```python
from build123d import *

# Parameters (mm, degrees)
SKETCH_1_W             = 140
SKETCH_1_H             = 80
EXTRUDE_1_DEPTH        = 2
SKETCH_2_W             = 5.5
SKETCH_2_H             = 5
SKETCH_2_H_2           = 3
EXTRUDE_2_DEPTH        = 12
SKETCH_3_W             = 30
SKETCH_3_H             = 80
CUT_EXTRUDE_1_DEPTH    = 3
SKETCH_4_W             = 36.4
SKETCH_4_H             = 15.6
SKETCH_4_W_2           = 30.4
SKETCH_4_H_2           = 9.6
EXTRUDE_3_DEPTH        = 18
SKETCH_5_W             = 10
SKETCH_5_H             = 27.4
CUT_EXTRUDE_2_DEPTH    = 20
SKETCH_6_W             = 1.3
SKETCH_6_H             = 9.6
EXTRUDE_4_DEPTH        = 3
SKETCH_8_W             = 10
SKETCH_8_H             = 6.6
CUT_EXTRUDE_3_DEPTH    = 40
PATTERN_LINEAR_1_COUNT = 2
PATTERN_LINEAR_1_PITCH = 40


with BuildPart() as part:
    # 草图1 → 凸台-拉伸1 (new body)
    with BuildSketch(Plane(origin=(0, 0, 0), x_dir=(0, 0, -1), z_dir=(1, 0, 0))):
        Rectangle(SKETCH_1_W, SKETCH_1_H)
    extrude(amount=EXTRUDE_1_DEPTH)

    # 草图2 → 凸台-拉伸2 (add)
    with BuildSketch(Plane(origin=(2, 0, 0), x_dir=(0, 0, -1), z_dir=(1, 0, 0))):
        with Locations((-24.05, -14.7)):
            Rectangle(SKETCH_2_W, SKETCH_2_H)
        with Locations((-52.75, -14.7)):
            Rectangle(SKETCH_2_W, SKETCH_2_H)
        with Locations((-24.05, -21.5)):
            Rectangle(SKETCH_2_W, SKETCH_2_H_2)
        with Locations((-52.75, 18.5)):
            Rectangle(SKETCH_2_W, SKETCH_2_H_2)
        with Locations((-24.05, 25.3)):
            Rectangle(SKETCH_2_W, SKETCH_2_H)
        with Locations((-52.75, -21.5)):
            Rectangle(SKETCH_2_W, SKETCH_2_H_2)
        with Locations((-24.05, 18.5)):
            Rectangle(SKETCH_2_W, SKETCH_2_H_2)
        with Locations((-52.75, 25.3)):
            Rectangle(SKETCH_2_W, SKETCH_2_H)
    extrude(amount=EXTRUDE_2_DEPTH)

    # 草图3 → 切除-拉伸1 (cut)
    with BuildSketch(Plane(origin=(2, 0, 0), x_dir=(0, 0, -1), z_dir=(1, 0, 0))):
        with Locations((55, 0)):
            Rectangle(SKETCH_3_W, SKETCH_3_H)
    extrude(amount=-CUT_EXTRUDE_1_DEPTH, mode=Mode.SUBTRACT)

    # 草图4 → 凸台-拉伸3 (add)
    with BuildSketch(Plane(origin=(2, 0, 0), x_dir=(0, 0, -1), z_dir=(1, 0, 0))):
        with Locations((18.9, -26.7)):
            Rectangle(SKETCH_4_W, SKETCH_4_H)
        with Locations((18.9, -26.7)):
            Rectangle(SKETCH_4_W_2, SKETCH_4_H_2, mode=Mode.SUBTRACT)
    extrude_3 = extrude(amount=EXTRUDE_3_DEPTH)

    # 草图5 → 切除-拉伸2 (cut)
    with BuildSketch(Plane.XZ.offset(34.5)):
        with Locations((7, -18.9)):
            Rectangle(SKETCH_5_W, SKETCH_5_H)
    cut_extrude_2 = extrude(amount=-CUT_EXTRUDE_2_DEPTH, mode=Mode.SUBTRACT)

    # 草图6 → 凸台-拉伸4 (add)
    with BuildSketch(Plane(origin=(2, 0, 0), x_dir=(0, 0, -1), z_dir=(1, 0, 0))):
        with Locations((4.35, -26.7)):
            Rectangle(SKETCH_6_W, SKETCH_6_H)
        with Locations((33.45, -26.7)):
            Rectangle(SKETCH_6_W, SKETCH_6_H)
    extrude_4 = extrude(amount=EXTRUDE_4_DEPTH)

    # 草图8 → 切除-拉伸3 (cut)
    with BuildSketch(Plane(origin=(0, 0, -37.1), x_dir=(-1, 0, 0), z_dir=(0, 0, -1))):
        with Locations((-7, -26.7)):
            Rectangle(SKETCH_8_W, SKETCH_8_H)
    cut_extrude_3 = extrude(amount=-CUT_EXTRUDE_3_DEPTH, mode=Mode.SUBTRACT)

    # 阵列(线性)1: 凸台-拉伸3, 切除-拉伸2, 凸台-拉伸4, 切除-拉伸3 ×2
    with Locations(*[(0, i * PATTERN_LINEAR_1_PITCH, 0) for i in range(1, PATTERN_LINEAR_1_COUNT)]):
        add(extrude_3)
        add(cut_extrude_2, mode=Mode.SUBTRACT)
        add(extrude_4)
        add(cut_extrude_3, mode=Mode.SUBTRACT)


solid = part.part
```
The listing builds one solid part. Answer for the finished solid, in the listing's coordinates (mm). A direction names the side the tool comes from. Round coordinates to 2 decimals unless told otherwise and drop trailing zeros. Order: outer loops, then holes, each group sorted by start corner. A loop starts at its lowest first (then second) coordinate and runs counter-clockwise, first axis right, second up. Notation, with made-up numbers: (16.5, 47) -> (32.5, 47) arc R10 ccw to (32.5, 64) -> close; hole circle Ø9 at (68, 27). An arc over 180 degrees is marked (long way). Answer as CSV lines item,"result".
Q1. Given pin 1 (8 mm diameter, centred on x = 10.5, y = -23, fed in from -Z); pin 2 (5 mm diameter, centred on x = 6.5, y = 2, fed in from +Z); pin 3 (6 mm diameter, centred on x = 5.5, z = 53.5, fed in from +Y); pin 4 (6 mm diameter, centred on x = 7.5, y = -20.5, fed in from +Z), each flat-ended and moving along its own axis, determine where each tip first touches the part or whether it passes through.
Computed values:
pin 1,"stops at z = -37.1"
pin 2,"passes through"
pin 3,"stops at y = 27.8"
pin 4,"stops at z = 55.5"
Q2. Which of the six approach directions +Z, -Z, +X, -X, +Y, -Y give full straight-line access (tool end or side, diameter ignored) to faces 4 (the flat face through (8, 22.8, 53)), 5 (the flat face through (14, 19, 53)), 6 (the flat face through (7, 16.6, -2))?
Computed values:
face 4,"+Z, -Z, +X"
face 5,"+Z, +X, +Y, -Y"
face 6,"+Z, -Z"
Q3. For a pull along Y with two mould halves and no side action, classify faces 1 (the flat face through (8, -15, 26.8)), 2 (the flat face through (7, -23.4, -35)), 3 (the flat face through (15, -34.5, -19)) as +Y half, -Y half, draft (parallel to the pull), parting line (faces both ways), or undercut.
Computed values:
face 1,"draft"
face 2,"undercut"
face 3,"-Y half"
Q4. A cutting plane is placed at B-B on z = -24. Determine the outline of the cut face in (x, y).
Computed values:
outline,"(0, -40) -> (2, -40) -> (2, 40) -> (0, 40) -> close; (12, -34.5) -> (20, -34.5) -> (20, -31.5) -> (12, -31.5) -> close; (12, -21.9) -> (20, -21.9) -> (20, -18.9) -> (12, -18.9) -> close; (12, 5.5) -> (20, 5.5) -> (20, 8.5) -> (12, 8.5) -> close; (12, 18.1) -> (20, 18.1) -> (20, 21.1) -> (12, 21.1) -> close"
Q5. A cutting plane is placed at A-A on x = 17.25. Determine the outline of the cut face in (y, z).
Computed values:
outline,"(-34.5, -37.1) -> (-18.9, -37.1) -> (-18.9, -0.7) -> (-34.5, -0.7) -> close; (5.5, -37.1) -> (21.1, -37.1) -> (21.1, -0.7) -> (5.5, -0.7) -> close; hole (-31.5, -34.1) -> (-21.9, -34.1) -> (-21.9, -3.7) -> (-31.5, -3.7) -> close; hole (8.5, -34.1) -> (18.1, -34.1) -> (18.1, -3.7) -> (8.5, -3.7) -> close"
Q6. A cutting plane is placed at C-C on y = 1.5. Determine the outline of the cut face in (x, z), plus the area to 3 significant figures.
Computed values:
outline,"(0, -40) -> (2, -40) -> (2, 70) -> (0, 70) -> close"
area,"220 mm^2"
Q7. A cutting plane is placed at D-D on x = 8.25. Give the number of separate pieces and of enclosed holes in the cut face, plus the area to 3 significant figures.
Computed values:
separate pieces,"16"
enclosed holes,"0"
area,"320 mm^2"
Q8. Consider line 1 (Y direction, x = 5.75, z = -1.5); line 2 (Z direction, x = 18, y = -29.5); line 3 (Y direction, x = 12.5, z = -10). Determine where each line is inside the solid, lowest interval first. Write a range as from..to.
Computed values:
line 1,"y = -34.5..-30, -23.4..-18.9, 5.5..10, 16.6..21.1"
line 2,"z = -37.1..-34.1, -3.7..-0.7"
line 3,"y = -34.5..-31.5, -21.9..-18.9, 5.5..8.5, 18.1..21.1"
